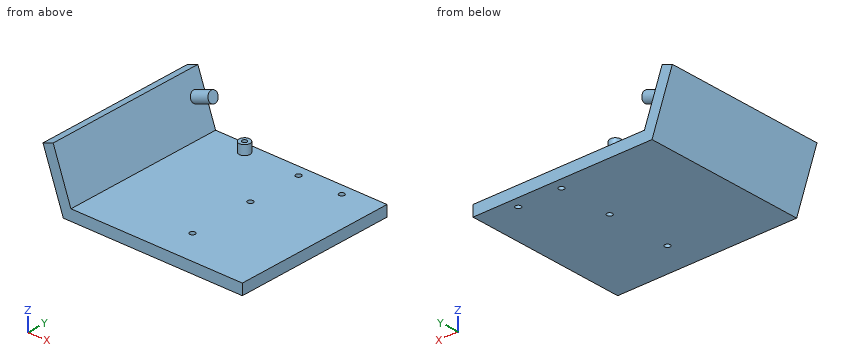
```python
from build123d import *

# Parameters (mm, degrees)
F1_DEPTH = 190.5
F2_R     = 3.175
F3_DEPTH = 12.701
F4_R     = 6.35
F5_DEPTH = 10.9982
F6_R     = 6.35
F7_DEPTH = 21.9964
F9_D     = 5.5118
F9_DEPTH = 12.7
F9_TIP   = 1.65591178


with BuildPart() as f1:
    # F0 (on Front) → F1 (new body)
    with BuildSketch(Plane.XZ):
        Polygon((-134.9451830515, 63.2994985103), (-111.0356246655, -3.3842598282), (99.5049753345, -3.3842598282), (99.5049753345, 9.3157401718), (-102.0975527369, 9.3157401718), (-122.9904038585, 67.5859019499), align=None)
    extrude(amount=F1_DEPTH)

    # F2 (on face) → F3 (cut, through all)
    with BuildSketch(Plane.XY.offset(9.3157401718)):
        with Locations((6.8430472631, -152.4)):
            Circle(F2_R)
        with Locations((6.8430472631, -76.2)):
            Circle(F2_R)
        with Locations((6.8430472631, -12.7)):
            Circle(F2_R)
        with Locations((57.6430472631, -12.7)):
            Circle(F2_R)
    extrude(amount=-F3_DEPTH, mode=Mode.SUBTRACT)

    # F4 (on face) → F5 (join)
    with BuildSketch(Plane.XY.offset(9.3157401718)):
        with Locations((-56.6569527369, -12.7)):
            Circle(F4_R)
    extrude(amount=F5_DEPTH)

    # F6 (on face) → F7 (join)
    with BuildSketch(Plane(origin=(-87.5074922841, 0, -31.375938431), x_dir=(0, 1, 0), z_dir=(0.9413211963, 0, 0.3375120819))):
        with Locations((-12.7, 79.7307893311)):
            Circle(F6_R)
    extrude(amount=F7_DEPTH)

    # F9
    with Locations(Plane.XY.offset(20.3139401718)):
        with Locations((-56.6569527369, -12.7)):
            Hole(F9_D / 2, depth=F9_DEPTH)
            with Locations((0, 0, -(F9_DEPTH + F9_TIP / 2))):  # 118° drill point
                Cone(0, F9_D / 2, F9_TIP, mode=Mode.SUBTRACT)


solid = f1.part
```
Geometry: final body of the model. Coordinates: model frame, mm. Coordinates: 2 decimals unless noted, no trailing zeros. Loops run counter-clockwise (first coordinate to the right, second up) from the corner with the lowest first, then second, coordinate; pieces in that order, holes last. Notation, with made-up numbers: M 33,-31.75 L 60,-31.75 A33 cw 60,5.25 Z; hole C -27,55 d5. An arc over 180 degrees is marked long. Put each result on its own line as item: value.
(1) Cut plane B-B on y = -144. Return the cut outline in (x, z).
Answer sheet:
outline: M -134.95,63.3 L -111.04,-3.38 L 99.5,-3.38 L 99.5,9.32 L -102.1,9.32 L -122.99,67.59 Z
(2) Cut plane C-C on x = -35. Return the cut outline in (y, z).
Answer sheet:
outline: M -190.5,-3.38 L 0,-3.38 L 0,9.32 L -190.5,9.32 Z
(3) Cut plane D-D on z = 23. Return the cut outline in (x, y).
Answer sheet:
outline: M -120.5,-190.5 L -107,-190.5 L -107,0 L -120.5,0 Z
(4) Material intervals for probe 1 along X at (y, z) = (-12, 15); probe 2 along Z at (x, y) = (81.5, -177); probe 3 along X at (y, z) = (-152.4, 4.75), sorted ascending.
Answer sheet:
probe 1: x = -117.63 to -104.14, -62.97 to -59.32, -53.99 to -50.35
probe 2: z = -3.38 to 9.32
probe 3: x = -113.95 to 3.67, 10.02 to 99.5
(5) Cut plane A-A on y = -76.2. Return the cut outline in (x, z).
Answer sheet:
outline: M -134.95,63.3 L -111.04,-3.38 L 3.67,-3.38 L 3.67,9.32 L -102.1,9.32 L -122.99,67.59 Z; M 10.02,-3.38 L 99.5,-3.38 L 99.5,9.32 L 10.02,9.32 Z
(6) First-contact query: pin 1 (4 mm diameter, centred on x = 6.84, y = -76.2, fed in from +Z); pin 2 (3 mm diameter, centred on y = -120, z = 27, fed in from +X); pin 3 (6.5 mm diameter, centred on x = -58, y = -13, fed in from +Z); pin 4 (12 mm diameter, centred on y = -59.5, z = 20, fed in from +X). Flat tips, straight axial feed; report the tip coordinate or a pass-through.
Answer sheet:
pin 1: passes through
pin 2: stops at x = -107.9
pin 3: stops at z = 20.31
pin 4: stops at x = -103.78
